Input: part model. Units: mm. Frame: model coordinates. Give positions to 0.01 mm unless a question says otherwise; leave off trailing zeros. Order: outer loops, then holes, each group sorted by start corner. A loop starts at its lowest first (then second) coordinate and runs counter-clockwise, first axis right, second up. Notation, with made-up numbers: (24.5, 24) -> (47.5, 24) arc R19 cw to (47.5, 61) -> close; hole circle Ø7 at (-15, 8.25). An arc over 180 degrees is marked (long way). Use a Markdown table: item, result. Add a question column.
from build123d import *

# Parameters (mm, degrees)
SKETCH1_W           = 120
SKETCH1_H           = 110
SKETCH1_R           = 1.5
SKETCH1_R_2         = 3.5
BOSS_EXTRUDE1_DEPTH = 1.5


with BuildPart() as part:
    # Sketch1 → Boss-Extrude1 (new body)
    with BuildSketch(Plane(origin=(0, 0, 0), x_dir=(1, 0, 0), z_dir=(0, 1, 0))):
        with Locations((60, 55)):
            Rectangle(SKETCH1_W, SKETCH1_H)
        with Locations(Location((5, 105, 0), (0, 0, 270))):
            Circle(SKETCH1_R, mode=Mode.SUBTRACT)
        with Locations(Location((115, 105, 0), (0, 0, 270))):
            Circle(SKETCH1_R, mode=Mode.SUBTRACT)
        with Locations(Location((115, 5, 0), (0, 0, 270))):
            Circle(SKETCH1_R, mode=Mode.SUBTRACT)
        with Locations(Location((5, 5, 0), (0, 0, 270))):
            Circle(SKETCH1_R, mode=Mode.SUBTRACT)
        with Locations(Location((100, 20, 0), (0, 0, 270))):
            Circle(SKETCH1_R_2, mode=Mode.SUBTRACT)
        with Locations(Location((20, 65, 0), (0, 0, 270))):
            Circle(SKETCH1_R_2, mode=Mode.SUBTRACT)
        with Locations(Location((20, 45, 0), (0, 0, 270))):
            Circle(SKETCH1_R_2, mode=Mode.SUBTRACT)
    extrude(amount=BOSS_EXTRUDE1_DEPTH)


solid = part.part
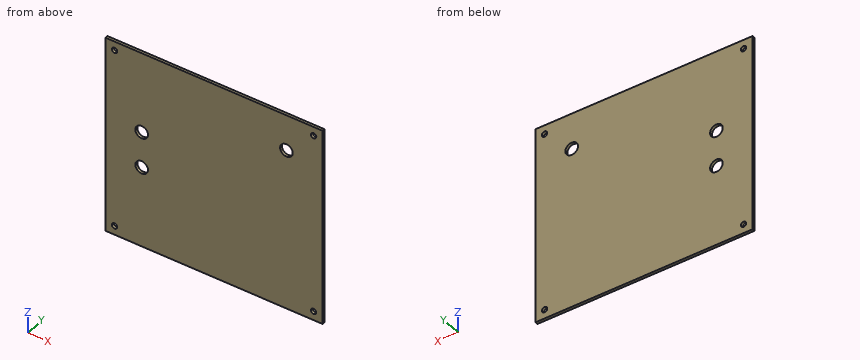
Q1. Section query C-C (z = -20). Return loops of the section in (x, y).
Q2. Section query B-B (x = 5). Return loops of the section in (y, z).
Q3. Section query A-A (z = -5). Return loops of the section in (x, y), plus the area to 3 significant figures.
Q4. Ray query, line 1 (X direction, y = 0.55, z = -5); line 2 (Z direction, x = 115, y = 0.85); line 3 (X direction, y = 1.1, z = -65). Return the intervals inside material, ascending.
Solution:
| question | item | result |
|---|---|---|
| 1 | outline | (0, 0) -> (96.5, 0) -> (96.5, 1.5) -> (0, 1.5) -> close; (103.5, 0) -> (120, 0) -> (120, 1.5) -> (103.5, 1.5) -> close |
| 2 | outline | (0, -110) -> (1.5, -110) -> (1.5, -106.5) -> (0, -106.5) -> close; (0, -103.5) -> (1.5, -103.5) -> (1.5, -6.5) -> (0, -6.5) -> close; (0, -3.5) -> (1.5, -3.5) -> (1.5, 0) -> (0, 0) -> close |
| 3 | outline | (0, 0) -> (3.5, 0) -> (3.5, 1.5) -> (0, 1.5) -> close; (6.5, 0) -> (113.5, 0) -> (113.5, 1.5) -> (6.5, 1.5) -> close; (116.5, 0) -> (120, 0) -> (120, 1.5) -> (116.5, 1.5) -> close |
| 3 | area | 171 mm² |
| 4 | line 1 | x = 0 to 3.5, 6.5 to 113.5, 116.5 to 120 |
| 4 | line 2 | z = -110 to -106.5, -103.5 to -6.5, -3.5 to 0 |
| 4 | line 3 | x = 0 to 16.5, 23.5 to 120 |
